```python
from build123d import *

# Parameters (mm, degrees)
BOSS_EXTRUDE1_DEPTH = 3
SKETCH2_R           = 1.23
CUT_EXTRUDE1_DEPTH  = 4


with BuildPart() as part:
    # Sketch1 → Boss-Extrude1 (new body)
    with BuildSketch(Plane.XY):
        Polygon((0, 0), (13, 0), (15, 2), (15, 20), (9, 20), (9, 3), (0, 3), align=None)
    extrude(amount=BOSS_EXTRUDE1_DEPTH)

    # Sketch2 → Cut-Extrude1 (cut, through all)
    with BuildSketch(Plane.XY.offset(3)):
        with Locations((12, 15)):
            Circle(SKETCH2_R)
        with Locations((12, 7)):
            Circle(SKETCH2_R)
    extrude(amount=-CUT_EXTRUDE1_DEPTH, mode=Mode.SUBTRACT)


solid = part.part
```
Can you work these out from the model? Positions are in its coordinate system, mm. A direction names the side the tool comes from. Coordinates: 2 decimals unless noted, no trailing zeros. Write each loop counter-clockwise with the first axis right and the second up, starting at its lowest first coordinate (ties: lowest second). Pieces come first, ordered by that corner, then holes. Notation, with made-up numbers: M 1.5,59.25 L 17.5,59.25 A22 cw 17.5,66.25 Z; hole C 74,47 d11. An arc over 180 degrees is marked long. Write item = value, one per line. Start each with the question number.
Q1. If we section it at D-D, the plane y = 17.25: Write out the boundary of the cut face in (x, z), then the cut area to 3 significant figures.
Q2. If we section it at C-C, the plane z = 2.5: Write out the boundary of the cut face in (x, y).
Q3. Thinking about a two-plate mould opening in X: for faces 3 (the face through (14, 1, 1)), 4 (the face through (13.136, 6.529, 1.521)), 5 (the face through (6, 0, 1)), which applies, released by +X, released by -X, zero draft, split by the parting line, or undercut?
Q4. I'm going to push flat-ended pins straight in: pin 1 (3 mm diameter, centred on x = 12, y = 15, fed in from -Z); pin 2 (0.9 mm diameter, centred on y = 11.5, z = 1.5, fed in from -X). Where does each tip first touch, or does it pass through?
Q5. If we section it at B-B, the plane y = 7: Write out the boundary of the cut face in (x, z).
Q6. If I drill on L1, parallel to Y at x = 12, z = 1.85; L2, parallel to X at y = 12.5, z = 0.6; L3, parallel to Y at x = 3.25, z = 1.3, over which ranges is the centre line in solid material (lowest first)? Write a range as [from, to].
Q7. If we section it at A-A, the plane x = 12: Write out the boundary of the cut face in (y, z).
Q8. On a 3-axis mill with a long thin cutter (end or side, diameter ignored), from which of +Z, -Z, +X, -X, +Y, -Y can I reach the whole of each face in a straight line? I mean faces 1 (the face through (5, 3, 1)), 2 (the face through (11, 8, 3)). Say none if no direction works.
Check sheet entries:
q1.outline = M 9,0 L 15,0 L 15,3 L 9,3 Z
q1.area = 18.0 mm²
q2.outline = M 0,0 L 13,0 L 15,2 L 15,20 L 9,20 L 9,3 L 0,3 Z; hole C 12,7 d2.46; hole C 12,15 d2.46
q3.face_3 = released by +X
q3.face_4 = undercut
q3.face_5 = zero draft
q4.pin_1 = 0
q4.pin_2 = 9
q5.outline = M 9,0 L 10.77,0 L 10.77,3 L 9,3 Z; M 13.23,0 L 15,0 L 15,3 L 13.23,3 Z
q6.L1 = [0, 5.77], [8.23, 13.77], [16.23, 20]
q6.L2 = [9, 15]
q6.L3 = [0, 3]
q7.outline = M 0,0 L 5.77,0 L 5.77,3 L 0,3 Z; M 8.23,0 L 13.77,0 L 13.77,3 L 8.23,3 Z; M 16.23,0 L 20,0 L 20,3 L 16.23,3 Z
q8.face_1 = +Z, -Z, -X, +Y
q8.face_2 = +Z, +X, -X, +Y, -Y
